```python
from build123d import *
from build123d import SkipClean  # not in build123d's __all__

# Parameters (mm, degrees)
F0_R          = 28.575
F1_DEPTH      = 64
F2_DEPTH      = 44
F4_W          = 114
F4_H          = 50
F5_DEPTH      = 22
F6_DEPTH      = 95.001
F6_DEPTH_BACK = 25
F7_R          = 11.1
F8_DEPTH      = 22.001
F10_DEPTH     = 10
F12_DEPTH     = 10


# Not quite as in the source:
# - after a boolean that leaves OpenCascade's solid faulty, fix() repairs it


with BuildPart() as f1:
    # F0 (on Front) → F1 (new body)
    with BuildSketch(Plane.XZ):
        with BuildLine():
            ThreePointArc((35.1425667816, -41), (49.0596504584, -22.5643678594), (54, 0))
            ThreePointArc((54, 0), (49.0596504584, 22.5643678594), (35.1425667816, 41))
            ThreePointArc((35.1425667816, 41), (-54, 0), (35.1425667816, -41))
        make_face()
        Circle(F0_R, mode=Mode.SUBTRACT)
    extrude(amount=F1_DEPTH)

    # F0 (on Front) → F2 (join)
    with BuildSketch(Plane.XZ):
        with BuildLine():
            ThreePointArc((35.1425667816, 41), (49.0596504584, 22.5643678594), (54, 0))
            ThreePointArc((54, 0), (49.0596504584, -22.5643678594), (35.1425667816, -41))
            Line((35.1425667816, -41), (209.1425667816, -41))
            Line((209.1425667816, -41), (209.1425667816, 41))
            Line((209.1425667816, 41), (35.1425667816, 41))
        make_face()
    extrude(amount=F2_DEPTH)

    # F4 (on face) → F5 (cut)
    with BuildSketch(Plane.XZ.offset(44)):
        with Locations((152.1425667816, 0)):
            Rectangle(F4_W, F4_H)
    extrude(amount=-F5_DEPTH, mode=Mode.SUBTRACT)

    # F3 (on face) → F6 (cut, two sides)
    with BuildSketch(Plane.XY.offset(41)) as f6_sk:
        Polygon((209.1425667816, -32), (197.1425667816, -44), (209.1425667816, -44), align=None)
    extrude(amount=-F6_DEPTH, mode=Mode.SUBTRACT)
    extrude(f6_sk.sketch, amount=F6_DEPTH_BACK, mode=Mode.SUBTRACT)

    # F7 (on face) → F8 (cut, through all)
    with BuildSketch(Plane.XZ.offset(22)):
        with Locations((124.1425667816, 0)):
            Circle(F7_R)
        with Locations((174.1425667816, 0)):
            Circle(F7_R)
    extrude(amount=-F8_DEPTH, mode=Mode.SUBTRACT)

    # F9 (on face) → F10 (join)
    with BuildSketch(Plane.XZ.offset(64)):
        with BuildLine():
            ThreePointArc((-23.6755279772, -16), (-28.575, 0), (-23.6755279772, 16))
            Line((-23.6755279772, 16), (-51.5751878329, 16))
            ThreePointArc((-51.5751878329, 16), (-54, 0), (-51.5751878329, -16))
            Line((-51.5751878329, -16), (-23.6755279772, -16))
        make_face()
    extrude(amount=F10_DEPTH)

    add(f1.part.fix(), mode=Mode.REPLACE)

    # F11 (on face) → F12 (join)
    with BuildSketch(Plane.XZ.offset(64)):
        with BuildLine():
            ThreePointArc((23.6755279772, 16), (28.575, 0), (23.6755279772, -16))
            Line((23.6755279772, -16), (51.5751878329, -16))
            ThreePointArc((51.5751878329, -16), (54, 0), (51.5751878329, 16))
            Line((51.5751878329, 16), (23.6755279772, 16))
        make_face()
    with SkipClean():  # cleaning this boolean's faces spoils the solid; the shape is the same uncleaned
        extrude(amount=F12_DEPTH)


solid = f1.part
```
Check sheet for the modelled part. Datum: model origin and axes. Units: mm. A direction names the side the tool comes from. Coordinates: 2 decimals unless noted, no trailing zeros. Order: outer loops, then holes, each group sorted by start corner. A loop starts at its lowest first (then second) coordinate and runs counter-clockwise, first axis right, second up. Notation, with made-up numbers: M 69,37.25 L 115,37.25 A18 ccw 115,54.25 Z; hole C -23.5,83 d11. An arc over 180 degrees is marked long. Write each question's results on one line, items separated by ' | '. Start each with the question number.
1. Go/stop test with flat-tipped pins: P1, Ø3, axis at x = -31, y = -66.5, coming from the +Z side; P2, Ø2, axis at x = 41, y = -15, coming from the -Z side; P3, Ø11.5, axis at x = 12, z = 33, coming from the -Y side. Record where each tip stops, or that it passes through.
2. Cross-section at B-B on y = -19.5. Record the cut outline in (x, z) (3 decimals).
3. Cross-section at A-A on x = 0. Record the cut outline in (y, z) (3 decimals), and give its area (3 significant figures).
4. Mould release check, pull along Z, two halves, no side actions. Record for faces 1 (the face through (184.73, -11.15, 3.33)), 2 (the face through (38, -69, 16)), 3 (the face through (115, -44, 28)), 4 (the face through (37, -69, -16)): +Z half, -Z half, draft (parallel to the pull), parting line (faces both ways), or undercut.
5. Cross-section at C-C on z = 5. Record the cut outline in (x, y).
6. Access from +Z, -Z, +X, -X, +Y, -Y to the whole of each face (thin tool, end or side, straight path). Record for faces 5 (the face through (121, -22, -41)), 6 (the face through (-38, -69, -16)), 7 (the face through (151, -22, 0)), 8 (the face through (123, -22, 41)).
7. Cross-section at D-D on x = 150. Record the cut outline in (y, z), and give its area (3 significant figures).
8. Material ranges on probe 1 along Z at (x, y) = (0, -20) (3 decimals); probe 2 along Z at (x, y) = (111, -33); probe 3 along X at (y, z) = (-36.5, 0) (3 decimals), recorded low to high.
Checks:
1) P1: stops at z = 16 | P2: stops at z = -41 | P3: stops at y = -64
2) outline: M 35.143,-41 L 209.143,-41 L 209.143,41 L 35.143,41 A54 ccw long Z; hole C 0,0 d57.15; hole C 124.143,0 d22.2; hole C 174.143,0 d22.2
3) outline: M -64,-54 L 0,-54 L 0,-28.575 L -64,-28.575 Z; M -64,28.575 L 0,28.575 L 0,54 L -64,54 Z | area: 3,250 mm²
4) face 1: undercut | face 2: +Z half | face 3: draft | face 4: -Z half
5) outline: M -53.77,-74 L -28.13,-74 L -28.13,0 L -53.77,0 Z; M 28.13,-74 L 53.77,-74 L 53.77,-44 L 95.14,-44 L 95.14,-22 L 114.23,-22 L 114.23,0 L 28.13,0 Z; M 134.05,-22 L 164.23,-22 L 164.23,0 L 134.05,0 Z; M 184.05,-22 L 209.14,-22 L 209.14,0 L 184.05,0 Z
6) face 5: -Z, +X, +Y, -Y | face 6: -Z, +X, -X, -Y | face 7: +X, -Y | face 8: +Z, +X, +Y, -Y
7) outline: M -44,-41 L 0,-41 L 0,41 L -44,41 L -44,25 L -22,25 L -22,-25 L -44,-25 Z | area: 2,510 mm²
8) probe 1: z = -54 to -28.575, 28.575 to 54 | probe 2: z = -41 to -25, 25 to 41 | probe 3: x = -54 to -28.575, 28.575 to 95.143
